Geometry check sheet. Reference: drawing and pictorial views, mm from the part's lowest x, y, z. A direction names the side the tool comes from. Give positions to 0.01 mm unless a question says otherwise; leave off trailing zeros. Loops run counter-clockwise (first coordinate to the right, second up) from the corner with the lowest first, then second, coordinate; pieces in that order, holes last. Notation, with made-up numbers: M 12,18 L 70,18 A33 ccw 70,54 Z; hole C 72.25,-16 d2. An arc over 180 degrees is marked long. Use CSV: the item, a comma, the result in double quotes.
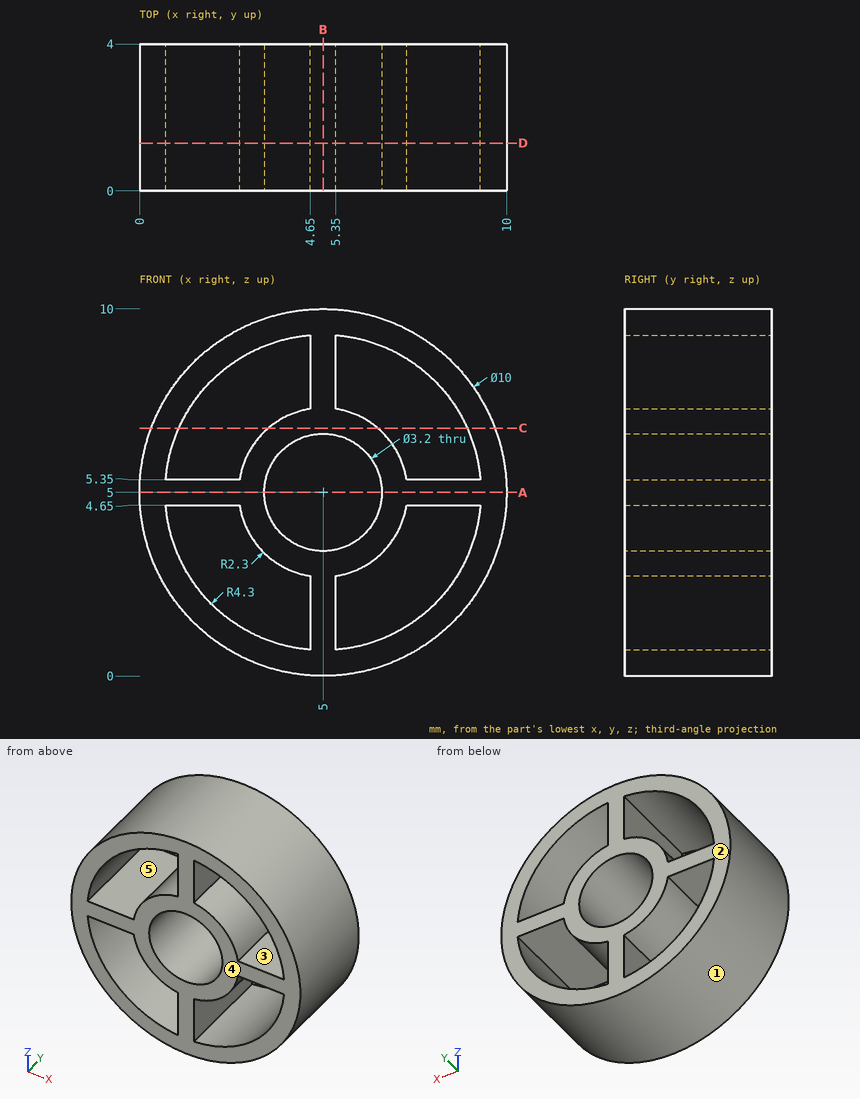
(1) Section check A-A on z = 5. Record the cut outline in (x, y), plus the area to 3 significant figures.
Calculated:
outline,"M 0,0 L 3.4,0 L 3.4,4 L 0,4 Z; M 6.6,0 L 10,0 L 10,4 L 6.6,4 Z"
area,"27.2 mm²"
(2) Scan lines: L1, parallel to X at y = 3.05, z = 5; L2, parallel to X at y = 2.6, z = 6; L3, parallel to Z at x = 8, y = 2.65. Record each from-to range of solid material in increasing order. Write a range as from..to.
Calculated:
L1,"x = 0..3.4, 6.6..10"
L2,"x = 0.1..0.82, 2.93..3.75, 6.25..7.07, 9.18..9.9"
L3,"z = 1..1.92, 4.65..5.35, 8.08..9"
(3) Section check C-C on z = 6.75. Record the cut outline in (x, y).
Calculated:
outline,"M 0.32,0 L 1.07,0 L 1.07,4 L 0.32,4 Z; M 3.51,0 L 6.49,0 L 6.49,4 L 3.51,4 Z; M 8.93,0 L 9.68,0 L 9.68,4 L 8.93,4 Z"
(4) Tool access check on the marked faces 4 and 5. Record the directions out of +Z, -Z, +X, -X, +Y, -Y that give a thin tool (end or side, any length) a straight path to the whole face; none if there is none.
Calculated:
face 4,"+Z, -Z, +X, -X, -Y"
face 5,"+Y, -Y"
(5) Section check D-D on y = 1.3. Record the cut outline in (x, z), plus the area to 3 significant figures.
Calculated:
outline,"C 5,5 d10; hole M 0.71,4.65 A4.3 ccw 4.65,0.71 L 4.65,2.73 A2.3 cw 2.73,4.65 Z; hole M 0.71,5.35 L 2.73,5.35 A2.3 cw 4.65,7.27 L 4.65,9.29 A4.3 ccw Z; hole C 5,5 d3.2; hole M 5.35,0.71 A4.3 ccw 9.29,4.65 L 7.27,4.65 A2.3 cw 5.35,2.73 Z; hole M 5.35,7.27 A2.3 cw 7.27,5.35 L 9.29,5.35 A4.3 ccw 5.35,9.29 Z"
area,"34.6 mm²"
(6) Depth check by flat-ended pin: pin 1 Ø1 at (y, z) = (1.5, 8.5) entering from +X; pin 2 Ø1.6 at (x, y) = (1.5, 3) entering from +Z; pin 3 Ø0.6 at (x, y) = (8.5, 2) entering from -Z. Enter the tip coordinate at first touch or a pass-through.
Calculated:
pin 1,"stops at x = 9"
pin 2,"stops at z = 9.21"
pin 3,"stops at z = 1.16"
(7) Mould release check, pull along Z, two halves, no side actions. Record for the marked faces 1, 2 and 3: released by +Z, released by -Z, zero draft, split by the parting line, or undercut.
Calculated:
face 1,"split by the parting line"
face 2,"zero draft"
face 3,"undercut"
(8) Section check B-B on x = 5. Record the cut outline in (y, z), plus the area to 3 significant figures.
Calculated:
outline,"M 0,0 L 4,0 L 4,3.4 L 0,3.4 Z; M 0,6.6 L 4,6.6 L 4,10 L 0,10 Z"
area,"27.2 mm²"
